Autodesk Inventor part; units mm, degrees
ref_plane "YZ Plane" through (0, 0, 0) normal (1, 0, 0) x (0, 1, 0)
ref_plane "XZ Plane" through (0, 0, 0) normal (0, 1, 0) x (-1, 0, 0)
ref_plane "XY Plane" through (0, 0, 0) normal (0, 0, 1) x (1, 0, 0)
sketch "スケッチ1" plane through (0, 0, 0) normal (0, 0, 1) x (1, 0, 0)
  line L0 (-4, 4.5) -> (4, 4.5)
  line L1 (4, 4.5) -> (4, -4.5)
  line L2 (4, -4.5) -> (-4, -4.5)
  line L3 (-4, -4.5) -> (-4, 4.5)
  line L4 (-4, 4.5) -> (4, -4.5) construction
  line L5 (4, 4.5) -> (-4, -4.5) construction
  point P0 (0, 0)
  dimension "d0" = 8
  dimension "d1" = 9
extrude "押し出し1" add sketch "スケッチ1" along normal blind 11
sketch "スケッチ2" plane through (0, 0, 11) normal (0, 0, 1) x (1, 0, 0)
  circle A0 centre (0, 1) radius 2
  circle A1 centre (0, 1) radius 1.3
  line L0 (-4, -4.5) -> (4, -4.5)
  point P0 (0, 0)
  dimension "d4" = 4
  dimension "d5" = 2.6
  dimension "d6" = 5.5
extrude "押し出し2" add sketch "スケッチ2" along normal blind 4
sketch "スケッチ3" plane through (-4, -4.5, 0) normal (0, -1, 0) x (1, 0, 0)
  line L0 (4.8, 9.85) -> (3.2, 9.85)
  line L1 (3.2, 9.85) -> (3.2, 9.55)
  line L2 (3.2, 9.55) -> (4.8, 9.55)
  line L3 (4.8, 9.55) -> (4.8, 9.85)
  line L4 (4.8, 9.85) -> (3.2, 9.55) construction
  line L5 (3.2, 9.85) -> (4.8, 9.55) construction
  line L6 (4.8, -0.15) -> (3.2, -0.15)
  line L7 (3.2, -0.15) -> (3.2, 0.15)
  line L8 (3.2, 0.15) -> (4.8, 0.15)
  line L9 (4.8, 0.15) -> (4.8, -0.15)
  line L10 (4.8, -0.15) -> (3.2, 0.15) construction
  line L11 (3.2, -0.15) -> (4.8, 0.15) construction
  line L12 (0, 11) -> (8, 11)
  line L13 (0.35, 2.3) -> (0.05, 2.3)
  line L14 (0.05, 2.3) -> (0.05, 0.7)
  line L15 (0.05, 0.7) -> (0.35, 0.7)
  line L16 (0.35, 0.7) -> (0.35, 2.3)
  line L17 (0.35, 2.3) -> (0.05, 0.7) construction
  line L18 (0.05, 2.3) -> (0.35, 0.7) construction
  point P0 (4, 0)
  point P1 (4, 9.7)
  point P2 (4, 9.7)
  point P3 (4, 0)
  point P4 (0.2, 1.5)
  dimension "d9" = 1.3
  dimension "d10" = 0.3
  dimension "d11" = 1.6
  dimension "d12" = 9.5
  dimension "d13" = 3.8
extrude "押し出し3" add sketch "スケッチ3" along normal blind 4
properties part number "Circuit_PhoneJack_HLA-2503D1l"
For this review, take the finished solid that the model builds, in its own axes (mm). A direction names the side the tool comes from. Round coordinates to 2 decimals unless told otherwise and drop trailing zeros. Order: outer loops, then holes, each group sorted by start corner. A loop starts at its lowest first (then second) coordinate and runs counter-clockwise, first axis right, second up.
Q1. Wall thickness on line 1 (Y direction, x = 0, z = 12.05); line 2 (Y direction, x = -0.5, z = 1.5); line 3 (Z direction, x = -0.25, y = -5.25): over which ranges is each line inside the solid? List them lowest first.
Findings below:
line 1: y = -1 to -0.3, 2.3 to 3
line 2: y = -4.5 to 4.5
line 3: z = -0.15 to 0.15, 9.55 to 9.85
Q2. We need section D-D, the plane y = 1. Give the boundary of the cut face in (x, z), plus the area to 3 significant figures.
Findings below:
outline: (-4, 0) - (4, 0) - (4, 11) - (2, 11) - (2, 15) - (1.3, 15) - (1.3, 11) - (-1.3, 11) - (-1.3, 15) - (-2, 15) - (-2, 11) - (-4, 11) - close
area: 93.6 mm2
Q3. We need section B-B, the plane z = 1.75. Give the boundary of the cut face in (x, y).
Findings below:
outline: (-4, -4.5) - (-3.95, -4.5) - (-3.95, -8.5) - (-3.65, -8.5) - (-3.65, -4.5) - (4, -4.5) - (4, 4.5) - (-4, 4.5) - close
Q4. We need section A-A, the plane y = -7. Give the boundary of the cut face in (x, z), plus the area to 3 significant figures.
Findings below:
outline: (-3.95, 0.7) - (-3.65, 0.7) - (-3.65, 2.3) - (-3.95, 2.3) - close; (-0.8, -0.15) - (0.8, -0.15) - (0.8, 0.15) - (-0.8, 0.15) - close; (-0.8, 9.55) - (0.8, 9.55) - (0.8, 9.85) - (-0.8, 9.85) - close
area: 1.44 mm2
Q5. We need section C-C, the plane x = 0. Give the boundary of the cut face in (y, z).
Findings below:
outline: (-8.5, -0.15) - (-4.5, -0.15) - (-4.5, 0) - (4.5, 0) - (4.5, 11) - (3, 11) - (3, 15) - (2.3, 15) - (2.3, 11) - (-0.3, 11) - (-0.3, 15) - (-1, 15) - (-1, 11) - (-4.5, 11) - (-4.5, 9.85) - (-8.5, 9.85) - (-8.5, 9.55) - (-4.5, 9.55) - (-4.5, 0.15) - (-8.5, 0.15) - close
Q6. Machinability: for faces 5 (the flat face through (-3.65, -6, 1)), 6 (the flat face through (0, -6, 0.15)), 7 (the flat face through (-1, -1, 11)), which of the approach directions +Z, -Z, +X, -X, +Y, -Y give a long, thin tool a straight path to every point of the face, cutting with its end or side? Answer none if there is none.
Findings below:
face 5: +Z, -Z, +X, -Y
face 6: +X, -X, -Y
face 7: +Z
Q7. Insertion check: P1, Ø0.8, axis at x = 0, y = -7, coming from the +Z side; P2, Ø4, axis at x = -1.5, z = 4.5, coming from the -Y side; P3, Ø1, axis at y = -6.5, z = 3, coming from the -X side; P4, Ø0.8, axis at y = -7.5, z = 1, coming from the -X side. Each pin has a flat end and moves straight along its axis. Give the tip position at first contact, or say it passes through.
Findings below:
P1: stops at z = 9.85
P2: stops at y = -4.5
P3: passes through
P4: stops at x = -3.95
Q8. Mouldability with a two-part tool opening along X and no side actions: class faces 1 (the cylindrical face through (1.908, 0.399, 12.972)), 2 (the flat face through (0, -6, 9.85)), 3 (the flat face through (0, 1, 11)), 4 (the flat face through (-3.95, -6, 2)) as pulls with the +X half, pulls with the -X half, needs draft (parallel to the pull), parting line crosses it, or undercut.
Findings below:
face 1: parting line crosses it
face 2: needs draft
face 3: undercut
face 4: pulls with the -X half
